For this review, take the finished solid that the model builds, in its own axes (mm). Round coordinates to 2 decimals unless told otherwise and drop trailing zeros. Write each loop counter-clockwise with the first axis right and the second up, starting at its lowest first coordinate (ties: lowest second). Pieces come first, ordered by that corner, then holes. Notation, with made-up numbers: M 42.5,35.25 L 81.5,35.25 A28 cw 81.5,56.25 Z; hole C 61,9 d2. An arc over 180 degrees is marked long. Write each question's results on one line, items separated by ' | '. Start each with the question number.
Autodesk Inventor part; units mm, degrees
ref_plane "YZ Plane" through (0, 0, 0) normal (1, 0, 0) x (0, 1, 0)
ref_plane "XZ Plane" through (0, 0, 0) normal (0, 1, 0) x (-1, 0, 0)
ref_plane "XY Plane" through (0, 0, 0) normal (0, 0, 1) x (1, 0, 0)
sketch "Sketch1" plane through (0, 0, 0) normal (0, 1, 0) x (-1, 0, 0)
  line L0 (0, 0) -> (0, -74.3966) construction
  circle A0 centre (0, 0) radius 5.08
  circle A1 centre (0, -74.3966) radius 5.08
  line L1 (5.08, 0) -> (5.08, -74.3966)
  line L2 (-5.08, -74.3966) -> (-5.08, 0)
  dimension "d0" = 74.3966
  dimension "d1" = 10.16
  dimension "d2" = 10.16
extrude "Extrusion1" add sketch "Sketch1" along normal blind 3.175
sketch "Sketch2" plane through (0, 3.175, 0) normal (0, 1, 0) x (1, 0, 0)
  arc A0 (5.08, 74.3966) -> (-5.08, 74.3966) centre (0, 74.3966) ccw
  point P0 (0, 0)
  point P1 (0, 0)
hole "Hole1" at (0, 3.175, 0) at (0, 3.175, -74.3966) direction (0, -1, 0) diameter 6.35 depth 25.4 tip angle 118
properties part number "linkage"
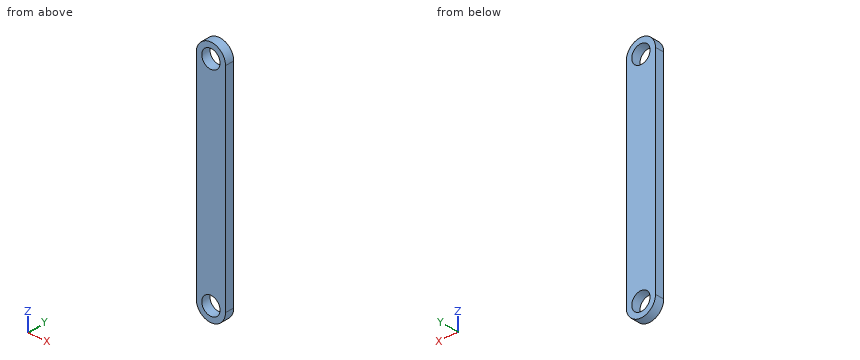
Item 1: For probe 1 along Z at (x, y) = (0, 1.65) (3 decimals); probe 2 along Z at (x, y) = (1, 0.6); probe 3 along X at (y, z) = (1.95, 0) (3 decimals), list the stretches that pass through material, from the lowest coordinate up.
Item 2: We need section B-B on y = 0.7. State the section outline as (x, z) points (3 decimals), then the cut area to 3 significant figures.
Item 3: We need section A-A on x = 0. State the section outline as (y, z) points (3 decimals), then the cut area to 3 significant figures.
Numbers:
1) probe 1: z = -79.477 to -77.572, -71.222 to -3.175, 3.175 to 5.08 | probe 2: z = -79.38 to -77.41, -71.38 to -3.01, 3.01 to 4.98 | probe 3: x = -5.08 to -3.175, 3.175 to 5.08
2) outline: M -5.08,-74.397 A5.08 ccw 5.08,-74.397 L 5.08,0 A5.08 ccw -5.08,0 Z; hole C 0,-74.397 d6.35; hole C 0,0 d6.35 | area: 774 mm^2
3) outline: M 0,-79.477 L 3.175,-79.477 L 3.175,-77.572 L 0,-77.572 Z; M 0,-71.222 L 3.175,-71.222 L 3.175,-3.175 L 0,-3.175 Z; M 0,3.175 L 3.175,3.175 L 3.175,5.08 L 0,5.08 Z | area: 228 mm^2
